from build123d import *

# Parameters (mm, degrees)
CYLINDER013_R     = 9.4
CYLINDER013_DEPTH = 6
CYLINDER014_R     = 16.75
CYLINDER014_DEPTH = 6
CYLINDER011_R     = 1
CYLINDER011_DEPTH = 100
CYLINDER006_R     = 9.4
CYLINDER006_DEPTH = 7
CYLINDER010_R     = 1.65
CYLINDER010_DEPTH = 100
CYLINDER009_R     = 1.65
CYLINDER009_DEPTH = 100
BOX003_W          = 50
BOX003_H          = 100
BOX003_DEPTH      = 100
CYLINDER012_R     = 23.5
CYLINDER012_DEPTH = 8
CYLINDER008_R     = 16.75
CYLINDER008_DEPTH = 43
CYLINDER007_R     = 16.75
CYLINDER007_DEPTH = 10


with BuildPart() as zylinder013:
    # Cylinder013 → Cylinder013 (new body)
    with BuildSketch(Plane.XY.offset(12)):
        Circle(CYLINDER013_R)
    extrude(amount=CYLINDER013_DEPTH)


with BuildPart() as cut006:
    # Cylinder014 → Cylinder014 (new body)
    with BuildSketch(Plane.XY.offset(12)):
        Circle(CYLINDER014_R)
    extrude(amount=CYLINDER014_DEPTH)

    # Cut006: cut Zylinder013
    add(zylinder013.part, mode=Mode.SUBTRACT)


with BuildPart() as zylinder011:
    # Cylinder011 → Cylinder011 (new body)
    with BuildSketch(Plane.XY.offset(5)):
        Circle(CYLINDER011_R)
    extrude(amount=CYLINDER011_DEPTH)


with BuildPart() as zylinder006:
    # Cylinder006 → Cylinder006 (new body)
    with BuildSketch(Plane.XY.offset(3)):
        Circle(CYLINDER006_R)
    extrude(amount=CYLINDER006_DEPTH)


with BuildPart() as zylinder010:
    # Cylinder010 → Cylinder010 (new body)
    with BuildSketch(Plane(origin=(-31, 16.75, 49.75), x_dir=(0, 0, -1), z_dir=(1, 0, 0))):
        Circle(CYLINDER010_R)
    extrude(amount=CYLINDER010_DEPTH)


with BuildPart() as compound003:
    # Cylinder009 → Cylinder009 (new body)
    with BuildSketch(Plane(origin=(-31, -19.75, 49.75), x_dir=(0, 0, -1), z_dir=(1, 0, 0))):
        Circle(CYLINDER009_R)
    extrude(amount=CYLINDER009_DEPTH)

    # Compound003: union Zylinder010
    add(zylinder010.part)


with BuildPart() as obj1:
    # Box003 → Box003 (new body)
    with BuildSketch(Plane(origin=(-2, -25, 0), x_dir=(1, 0, 0), z_dir=(0, 0, 1))):
        with Locations((25, 50)):
            Rectangle(BOX003_W, BOX003_H)
    extrude(amount=BOX003_DEPTH)


with BuildPart() as zylinder012:
    # Cylinder012 → Cylinder012 (new body)
    with BuildSketch(Plane.XY.offset(45)):
        Circle(CYLINDER012_R)
    extrude(amount=CYLINDER012_DEPTH)


with BuildPart() as cut004:
    # Cylinder008 → Cylinder008 (new body)
    with BuildSketch(Plane.XY.offset(10)):
        Circle(CYLINDER008_R)
    extrude(amount=CYLINDER008_DEPTH)

    # Fusion: union Zylinder012
    add(zylinder012.part)

    # Cut003: cut obj1
    add(obj1.part, mode=Mode.SUBTRACT)

    # Cut004: cut Compound003
    add(compound003.part, mode=Mode.SUBTRACT)


with BuildPart() as cut007:
    # Cylinder007 → Cylinder007 (new body)
    with BuildSketch(Plane.XY.offset(10)):
        Circle(CYLINDER007_R)
    extrude(amount=CYLINDER007_DEPTH)

    # Fusion001: union Zylinder006, Cut004
    add(zylinder006.part)
    add(cut004.part)

    # Cut005: cut Zylinder011
    add(zylinder011.part, mode=Mode.SUBTRACT)

    # Cut007: cut Cut006
    add(cut006.part, mode=Mode.SUBTRACT)


solid = cut007.part
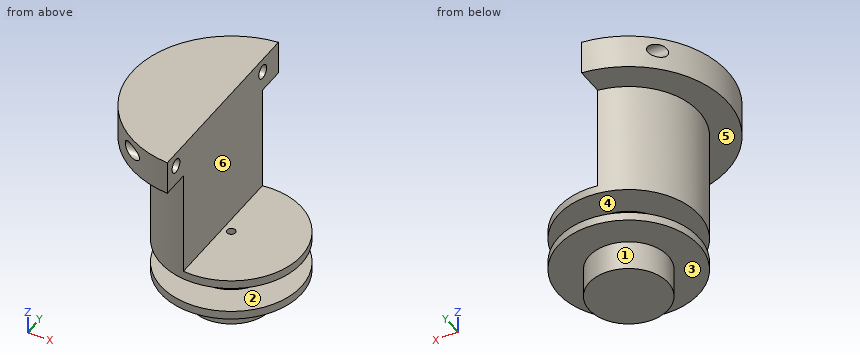
For this review, take the finished solid that the model builds, in its own axes (mm). Face numbers are marked on the shaded views. A direction names the side the tool comes from. Round coordinates to 2 decimals unless told otherwise and drop trailing zeros. Loops run counter-clockwise (first coordinate to the right, second up) from the corner with the lowest first, then second, coordinate; pieces in that order, holes last. Notation, with made-up numbers: (60.5, 38.25) - (87.5, 38.25) arc R18 cw to (87.5, 72.25) - close; hole circle Ø1 at (7.25, -19). An arc over 180 degrees is marked (long way). Answer as CSV lines item,"result".
(1) Tool access review of the marked faces 4, 5 and 6: name each direction out of +Z, -Z, +X, -X, +Y, -Y from which nothing blocks a thin tool from reaching the whole face with its end or side.
Checked values:
face 4,"none"
face 5,"-Z, -X"
face 6,"+Z, +X, +Y, -Y"
(2) Consider section B-B on y = 0. Give the boundary of the cut face in (x, z), then the cut area to 3 significant figures.
Checked values:
outline,"(-23.5, 45) - (-16.75, 45) - (-16.75, 18) - (-9.4, 18) - (-9.4, 12) - (-16.75, 12) - (-16.75, 10) - (-9.4, 10) - (-9.4, 3) - (9.4, 3) - (9.4, 10) - (16.75, 10) - (16.75, 12) - (9.4, 12) - (9.4, 18) - (16.75, 18) - (16.75, 20) - (1, 20) - (1, 5) - (-1, 5) - (-1, 20) - (-2, 20) - (-2, 53) - (-23.5, 53) - close"
area,"889 mm2"
(3) Mouldability with a two-part tool opening along Z and no side actions: class the marked faces 1, 2 and 3 as +Z half, -Z half, draft (parallel to the pull), parting line (faces both ways), or undercut.
Checked values:
face 1,"draft"
face 2,"undercut"
face 3,"-Z half"
(4) Wall thickness on line 1 (Y direction, x = -5, z = 49); line 2 (Y direction, x = 0, z = 11.75); line 3 (Y direction, x = -5.75, z = 49.75): over which ranges is each line inside the solid? List them lowest first.
Checked values:
line 1,"y = -22.96 to -21.22, -18.28 to 15.28, 18.22 to 22.96"
line 2,"y = -16.75 to -1, 1 to 16.75"
line 3,"y = -22.79 to -21.4, -18.1 to 15.1, 18.4 to 22.79"
(5) Consider section C-C on x = 12. Give the boundary of the cut face in (y, z).
Checked values:
outline,"(-11.69, 10) - (11.69, 10) - (11.69, 12) - (-11.69, 12) - close; (-11.69, 18) - (11.69, 18) - (11.69, 20) - (-11.69, 20) - close"
(6) Consider section D-D on y = -10.5. Give the boundary of the cut face in (x, z).
Checked values:
outline,"(-21.02, 45) - (-13.05, 45) - (-13.05, 18) - (13.05, 18) - (13.05, 20) - (-2, 20) - (-2, 53) - (-21.02, 53) - close; (-13.05, 10) - (13.05, 10) - (13.05, 12) - (-13.05, 12) - close"
(7) Insertion check: P1, Ø1.5, axis at x = -13.5, z = 23.5, coming from the +Y side; P2, Ø9.5, axis at x = 5, y = -0.5, coming from the +Z side; P3, Ø5.5, axis at y = 16.75, z = 49.75, coming from the +X side; P4, Ø2.5, axis at y = -19.75, z = 49.75, coming from the -X side. Each pin has a flat end and moves straight along its axis. Give the tip position at first contact, or say it passes through.
Checked values:
P1,"stops at y = 10.86"
P2,"stops at z = 20"
P3,"stops at x = -2"
P4,"passes through"
(8) Consider section A-A on z = 49.75. Give the boundary of the cut face in (x, y), then the cut area to 3 significant figures.
Checked values:
outline,"(-18.01, 15.1) arc R23.5 ccw to (-14.99, -18.1) - (-2, -18.1) - (-2, 15.1) - close; (-14.62, 18.4) - (-2, 18.4) - (-2, 23.41) arc R23.5 ccw to start; (-9.71, -21.4) arc R23.5 ccw to (-2, -23.41) - (-2, -21.4) - close"
area,"691 mm2"
